from build123d import *
from OCP.BRepFilletAPI import BRepFilletAPI_MakeFillet

# Parameters (mm, degrees)
SKETCH_1_W          = 58
SKETCH_1_H          = 10
EXTRUDE_1_DEPTH     = 3
SKETCH_3_W          = 10
SKETCH_3_H          = 3
CUT_EXTRUDE_2_DEPTH = 30.580398915
EXTRUDE_2_DEPTH     = 3
SKETCH_5_R          = 1
SKETCH_5_R_2        = 1.35
CUT_EXTRUDE_3_DEPTH = 39.082148049
CUT_EXTRUDE_5_DEPTH = 39.082148049
FILLET_1_R          = 1
FILLET_2_R          = 2
FILLET_3_R1         = 5
FILLET_3_R2         = 8


with BuildPart() as part:
    # 草图1 → 凸台-拉伸1 (new body)
    with BuildSketch(Plane(origin=(0, 0, 0), x_dir=(1, 0, 0), z_dir=(0, 1, 0))):
        Rectangle(SKETCH_1_W, SKETCH_1_H)
    extrude(amount=EXTRUDE_1_DEPTH)

    # 草图3 → 切除-拉伸2 (cut, through all)
    with BuildSketch(Plane.XZ):
        with Locations((-19, 0)):
            Rectangle(SKETCH_3_W, SKETCH_3_H)
        with Locations((1, 0)):
            Rectangle(SKETCH_3_W, SKETCH_3_H)
        with Locations((21, 0)):
            Rectangle(SKETCH_3_W, SKETCH_3_H)
    extrude(amount=-CUT_EXTRUDE_2_DEPTH, mode=Mode.SUBTRACT)

    # 草图9 → 凸台-拉伸2 (add)
    with BuildSketch(Plane(origin=(0, 3, 0), x_dir=(1, 0, 0), z_dir=(0, 1, 0))):
        with BuildLine():
            Line((29, 24.5), (29, 5))
            Line((29, 5), (22, 5))
            Line((22, 5), (16.19691326, 5))
            ThreePointArc((16.19691326, 5), (17.182388504, 5.830180852), (16.531618392, 6.942322914))
            Line((16.531618392, 6.942322914), (0, 12.814213999))
            Line((0, 12.814213999), (-21.639361843, 5))
            Line((-21.639361843, 5), (-29, 5))
            Line((-29, 5), (25, 24.5))
            Line((25, 24.5), (29, 24.5))
        make_face()
        Polygon((25, 21.841991777), (25, 8.5), (22, 8.5), (4.886202736, 14.578676098), align=None, mode=Mode.SUBTRACT)
    extrude(amount=-EXTRUDE_2_DEPTH)

    # 草图5 → 切除-拉伸3 (cut, through all)
    with BuildSketch(Plane.XZ):
        with Locations((-23, 1.5)):
            Circle(SKETCH_5_R)
        with Locations((-15, 1.5)):
            Circle(SKETCH_5_R)
        with Locations((-15, -1.5)):
            Circle(SKETCH_5_R)
        with Locations((-23, -1.5)):
            Circle(SKETCH_5_R)
        with Locations((-3, -1.5)):
            Circle(SKETCH_5_R)
        with Locations((5, -1.5)):
            Circle(SKETCH_5_R)
        with Locations((-3, 1.5)):
            Circle(SKETCH_5_R)
        with Locations((5, 1.5)):
            Circle(SKETCH_5_R)
        with Locations(Location((22, -5.5, 0), (0, 0, 270))):
            Circle(SKETCH_5_R_2)
        with Locations((25, -1.5)):
            Circle(SKETCH_5_R)
        with Locations((17, -1.5)):
            Circle(SKETCH_5_R)
        with Locations((17, 1.5)):
            Circle(SKETCH_5_R)
        with Locations((25, 1.5)):
            Circle(SKETCH_5_R)
    extrude(amount=-CUT_EXTRUDE_3_DEPTH, mode=Mode.SUBTRACT)

    # 草图8 → 切除-拉伸5 (cut, through all)
    with BuildSketch(Plane(origin=(0, 3, 0), x_dir=(1, 0, 0), z_dir=(0, 1, 0))):
        with BuildLine():
            Line((6.1, -1.5), (6.1, 1.5))
            ThreePointArc((6.1, 1.5), (5.050051841, 2.598860689), (3.904554885, 1.6))
            Line((3.904554885, 1.6), (-1.904554885, 1.6))
            ThreePointArc((-1.904554885, 1.6), (-3.050051841, 2.598860689), (-4.1, 1.5))
            Line((-4.1, 1.5), (-4.1, -1.5))
            ThreePointArc((-4.1, -1.5), (-3.050051841, -2.598860689), (-1.904554885, -1.6))
            Line((-1.904554885, -1.6), (3.904554885, -1.6))
            ThreePointArc((3.904554885, -1.6), (5.050051841, -2.598860689), (6.1, -1.5))
        make_face()
        with BuildLine():
            Line((-16.095445115, -1.6), (-21.904554885, -1.6))
            ThreePointArc((-21.904554885, -1.6), (-23.050051841, -2.598860689), (-24.1, -1.5))
            Line((-24.1, -1.5), (-24.1, 1.5))
            ThreePointArc((-24.1, 1.5), (-23.050051841, 2.598860689), (-21.904554885, 1.6))
            Line((-21.904554885, 1.6), (-16.095445115, 1.6))
            ThreePointArc((-16.095445115, 1.6), (-14.949948159, 2.598860689), (-13.9, 1.5))
            Line((-13.9, 1.5), (-13.9, -1.5))
            ThreePointArc((-13.9, -1.5), (-14.949948159, -2.598860689), (-16.095445115, -1.6))
        make_face()
        with BuildLine():
            Line((23.904554885, -1.6), (18.095445115, -1.6))
            ThreePointArc((18.095445115, -1.6), (16.949948159, -2.598860689), (15.9, -1.5))
            Line((15.9, -1.5), (15.9, 1.5))
            ThreePointArc((15.9, 1.5), (16.949948159, 2.598860689), (18.095445115, 1.6))
            Line((18.095445115, 1.6), (23.904554885, 1.6))
            ThreePointArc((23.904554885, 1.6), (25.050051841, 2.598860689), (26.1, 1.5))
            Line((26.1, 1.5), (26.1, -1.5))
            ThreePointArc((26.1, -1.5), (25.050051841, -2.598860689), (23.904554885, -1.6))
        make_face()
    extrude(amount=-CUT_EXTRUDE_5_DEPTH, mode=Mode.SUBTRACT)

    # 圆角1
    fillet_1_edges = [part.edges().sort_by_distance(p)[0] for p in [
        (-21.639361843, 1.5, -5),
        (25, 1.5, -21.841991777),
        (25, 1.5, -8.5),
        (4.886202736, 1.5, -14.578676098),
    ]]
    fillet(fillet_1_edges, radius=FILLET_1_R)

    # 圆角2
    fillet_2_edges = [part.edges().sort_by_distance(p)[0] for p in [
        (29, 1.5, -24.5),
        (29, 1.5, 5),
        (-29, 1.5, 5),
        (-29, 1.5, -5),
    ]]
    fillet(fillet_2_edges, radius=FILLET_2_R)

    # 圆角3: one fillet with a radius per group of edges: ONE call of the kernel's fillet builder (fillet() takes one radius for all edges)
    fillet_3_edges_1 = [part.edges().sort_by_distance(p)[0] for p in [
        (0, 1.5, -12.814213999),
        (25, 1.5, -24.5),
    ]]
    fillet_3_edges_2 = [part.edges().sort_by_distance(p)[0] for p in [
        (22, 1.5, -8.5),
    ]]
    fillet_3 = BRepFilletAPI_MakeFillet(part.part.solid().wrapped)
    for e in fillet_3_edges_1:
        fillet_3.Add(FILLET_3_R1, e.wrapped)
    for e in fillet_3_edges_2:
        fillet_3.Add(FILLET_3_R2, e.wrapped)
    add(Compound.cast(fillet_3.Shape()), mode=Mode.REPLACE)


solid = part.part
Can you work these out from the model? Positions are in its coordinate system, mm. A direction names the side the tool comes from. Coordinates: 2 decimals unless noted, no trailing zeros. Write each loop counter-clockwise with the first axis right and the second up, starting at its lowest first coordinate (ties: lowest second). Pieces come first, ordered by that corner, then holes. Notation, with made-up numbers: (-4, -8.75) -> (5, -8.75) arc R20 ccw to (5, 14.25) -> close; hole circle Ø10 at (33, 84). An arc over 180 degrees is marked (long way). Answer as CSV lines item,"result".
1) If we section it at B-B on x = 13.5: Please give me the cut outline in (y, z).
Check result:
outline,"(0, -20.35) -> (3, -20.35) -> (3, -17.69) -> (0, -17.69) -> close; (0, -11.52) -> (3, -11.52) -> (3, -8.02) -> (0, -8.02) -> close; (0, -5) -> (3, -5) -> (3, 5) -> (0, 5) -> close"
2) On a 3-axis mill with a long thin cutter (end or side, diameter ignored), from which of +Z, -Z, +X, -X, +Y, -Y can I reach the whole of each face in a straight line? I mean faces 4 (the cylindrical face through (-23.074, 1.521, -2.598)), 5 (the flat face through (-29, 1, 0)). Say none if no direction works.
Check result:
face 4,"+Y, -Y"
face 5,"+Z, -Z, -X, +Y, -Y"
3) If we section it at A-A on x = -20: Please give me the cut outline in (y, z), then the cut area to 4 significant figures.
Check result:
outline,"(0, -8.25) -> (3, -8.25) -> (3, -1.6) -> (0, -1.6) -> close; (0, 1.6) -> (3, 1.6) -> (3, 5) -> (0, 5) -> close"
area,"30.15 mm²"
4) Will these pins go through, and if not, where does the flat tip stop? P1, Ø0.9, axis at x = 22, y = 1.5, coming from the -Z side; P2, Ø0.9, axis at x = -19.5, y = 1.5, coming from the -Z side; P3, Ø0.5, axis at x = 23.5, y = 1, coming from the -Z side.
Check result:
P1,"z = -23.58"
P2,"z = -8.59"
P3,"z = -24.05"
5) If we section it at C-C on z = -17.5: Please give me the cut outline in (x, y), then the cut area to 3 significant figures.
Check result:
outline,"(5.62, 0) -> (12.98, 0) -> (12.98, 3) -> (5.62, 3) -> close; (25, 0) -> (29, 0) -> (29, 3) -> (25, 3) -> close"
area,"34.1 mm²"
6) If I drill on line 1 (Z direction, x = 15.5, y = 1.05); line 2 (Z direction, x = 8, y = 0.2); line 3 (Z direction, x = -18.5, y = 2.35), over which ranges is the centre line in solid material (lowest first)? Write a range as from..to.
Check result:
line 1,"-21.07..-18.41, -10.81..-7.31, -5..5"
line 2,"-18.36..-15.7, -13.47..-9.97, -5..5"
line 3,"-8.79..-1.6, 1.6..5"
7) If we section it at D-D on y = 2.3: Count the separate pieces of the cut face and the enclosed holes in it, then the cut area to 3 significant figures.
Check result:
separate pieces,"1"
enclosed holes,"6"
area,"755 mm²"
8) If we mould it in two halves opening along Z, with no side actions, what happens to faces 1 (the flat face through (-2.11, 1.52, -14.71)), 2 (the cylindrical face through (28.43, 1.52, 4.4)), 3 (the cylindrical face through (24.715, 1.479, -8.801))? For each: +Z half, -Z half, draft (parallel to the pull), parting line (faces both ways), or undercut.
Check result:
face 1,"-Z half"
face 2,"+Z half"
face 3,"undercut"
